Read the model definition and answer for the solid it produces. Units are mm, in the model's axes. Face numbers are marked on the shaded views. A direction names the side the tool comes from. Round coordinates to 2 decimals unless told otherwise and drop trailing zeros. Loops run counter-clockwise (first coordinate to the right, second up) from the corner with the lowest first, then second, coordinate; pieces in that order, holes last. Notation, with made-up numbers: (-20, 36) -> (13, 36) arc R13 ccw to (13, 50) -> close; hole circle Ø3 at (-3.5, 35.5). An arc over 180 degrees is marked (long way). Put each result on its own line as item: value.
from build123d import *

# Parameters (mm, degrees)
SKETCH1_W           = 100
SKETCH1_H           = 62
BOSS_EXTRUDE1_DEPTH = 20
SKETCH2_W           = 37
SKETCH2_H           = 62
BOSS_EXTRUDE2_DEPTH = 24
CUT_EXTRUDE2_DEPTH  = 12
SKETCH4_R           = 5
CUT_EXTRUDE3_DEPTH  = 33
SKETCH5_R           = 3
CUT_EXTRUDE4_DEPTH  = 20
SKETCH12_R          = 3
CUT_EXTRUDE12_DEPTH = 20
CUT_EXTRUDE13_DEPTH = 21
SKETCH14_W          = 6
SKETCH14_H          = 50
CUT_EXTRUDE14_DEPTH = 101


with BuildPart() as part:
    # Sketch1 → Boss-Extrude1 (new body)
    with BuildSketch(Plane.XY):
        Rectangle(SKETCH1_W, SKETCH1_H)
    extrude(amount=BOSS_EXTRUDE1_DEPTH)

    # Sketch2 → Boss-Extrude2 (add)
    with BuildSketch(Plane.XY.offset(20)):
        with Locations((-31.5, 0)):
            Rectangle(SKETCH2_W, SKETCH2_H)
    extrude(amount=BOSS_EXTRUDE2_DEPTH)

    # Sketch3 → Cut-Extrude2 (cut)
    with BuildSketch(Plane.XY.offset(44)):
        Polygon((-50, 12), (-13, 18.5), (-13, -18.5), (-50, -12), align=None)
    extrude(amount=-CUT_EXTRUDE2_DEPTH, mode=Mode.SUBTRACT)

    # Sketch4 → Cut-Extrude3 (cut, through all)
    with BuildSketch(Plane.XY.offset(32)):
        with Locations((-33, 0)):
            Circle(SKETCH4_R)
    extrude(amount=-CUT_EXTRUDE3_DEPTH, mode=Mode.SUBTRACT)

    # Sketch5 → Cut-Extrude4 (cut)
    with BuildSketch(Plane.XY.offset(44)):
        with Locations((-38, 22)):
            Circle(SKETCH5_R)
    extrude(amount=-CUT_EXTRUDE4_DEPTH, mode=Mode.SUBTRACT)

    # Sketch12 → Cut-Extrude12 (cut)
    with BuildSketch(Plane.XY.offset(44)):
        with Locations((-38, -22)):
            Circle(SKETCH12_R)
    extrude(amount=-CUT_EXTRUDE12_DEPTH, mode=Mode.SUBTRACT)

    # Sketch13 → Cut-Extrude13 (cut, through all)
    with BuildSketch(Plane.XY.offset(20)):
        with BuildLine():
            Line((8.5, 8), (28.5, 8))
            ThreePointArc((28.5, 8), (36.5, 0), (28.5, -8))
            Line((28.5, -8), (8.5, -8))
            ThreePointArc((8.5, -8), (0.5, 0), (8.5, 8))
        make_face()
    extrude(amount=-CUT_EXTRUDE13_DEPTH, mode=Mode.SUBTRACT)

    # Sketch14 → Cut-Extrude14 (cut, through all)
    with BuildSketch(Plane(origin=(50, 0, 0), x_dir=(0, 0, -1), z_dir=(1, 0, 0))):
        with Locations((-3, 0)):
            Rectangle(SKETCH14_W, SKETCH14_H)
    extrude(amount=-CUT_EXTRUDE14_DEPTH, mode=Mode.SUBTRACT)


solid = part.part
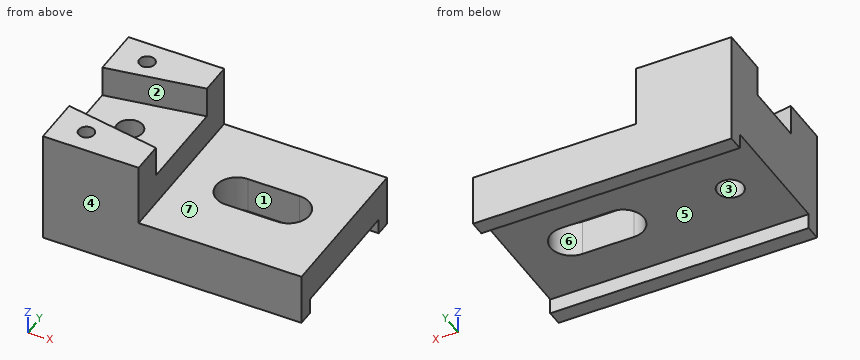
Item 1: The part is cut by section A-A (z = 4). Determine the outline of the cut face in (x, y).
Derived:
outline: (-50, -31) -> (50, -31) -> (50, -25) -> (-50, -25) -> close; (-50, 25) -> (50, 25) -> (50, 31) -> (-50, 31) -> close
Item 2: Flat-ended cylindrical pins translate along their axes: pin 1 Ø5 at (x, y) = (-38, 22) entering from -Z; pin 2 Ø1.5 at (y, z) = (23.5, 26) entering from +X; pin 3 Ø18.5 at (x, y) = (15.5, 15) entering from +Z; pin 4 Ø10 at (x, z) = (2, 22) entering from +Y. Find the tip coordinate at first contact, or state that the pin passes through.
Derived:
pin 1: stops at z = 6
pin 2: stops at x = -13
pin 3: stops at z = 20
pin 4: stops at y = 31
Item 3: The part is cut by section D-D (x = -1). Determine the outline of the cut face in (y, z).
Derived:
outline: (-31, 0) -> (-25, 0) -> (-25, 6) -> (25, 6) -> (25, 0) -> (31, 0) -> (31, 20) -> (-31, 20) -> close
Item 4: The part is cut by section B-B (y = 0). Determine the outline of the cut face in (x, z).
Derived:
outline: (-50, 6) -> (-38, 6) -> (-38, 32) -> (-50, 32) -> close; (-28, 6) -> (0.5, 6) -> (0.5, 20) -> (-13, 20) -> (-13, 32) -> (-28, 32) -> close; (36.5, 6) -> (50, 6) -> (50, 20) -> (36.5, 20) -> close
Item 5: Which of the six approach directions +Z, -Z, +X, -X, +Y, -Y give full straight-line access (tool end or side, diameter ignored) to the marked faces 5, 6 and 7?
Derived:
face 5: -Z, +X, -X
face 6: +Z, -Z
face 7: +Z, +X, +Y, -Y
Item 6: Find the intervals of material crossed by line 1 along Y through (x, z) = (-3, 3); line 2 along Z through (x, y) = (-11, -7.5); line 3 along Z through (x, y) = (-34.5, -8.5), in increasing order.
Derived:
line 1: y = -31 to -25, 25 to 31
line 2: z = 6 to 20
line 3: z = 6 to 32
Item 7: For a pull along X with two mould halves and no side action, classify the marked faces 1, 2, 3 and 4 as pulls with the +X half, pulls with the -X half, needs draft (parallel to the pull), parting line crosses it, or undercut.
Derived:
face 1: undercut
face 2: pulls with the +X half
face 3: undercut
face 4: needs draft
Item 8: The part is cut by section C-C (z = 34). Determine the outline of the cut face in (x, y).
Derived:
outline: (-50, -31) -> (-13, -31) -> (-13, -18.5) -> (-50, -12) -> close; (-50, 12) -> (-13, 18.5) -> (-13, 31) -> (-50, 31) -> close; hole circle Ø6 at (-38, -22); hole circle Ø6 at (-38, 22)
